from build123d import *

# Parameters (mm, degrees)
ESBO_O1_W                = 20
ESBO_O1_H                = 20
RESSALTO_EXTRUS_O3_DEPTH = 2
CORTE_EXTRUS_O5_DEPTH    = 29.354893758


with BuildPart() as part:
    # Esboço1 → Ressalto-extrusão3 (new body)
    with BuildSketch(Plane(origin=(0, 0, 0), x_dir=(1, 0, 0), z_dir=(0, 1, 0))):
        with Locations((10, 10)):
            Rectangle(ESBO_O1_W, ESBO_O1_H)
    extrude(amount=RESSALTO_EXTRUS_O3_DEPTH)

    # Esboço5 → Corte-extrusão5 (cut, through all)
    with BuildSketch(Plane(origin=(0, 2, 0), x_dir=(1, 0, 0), z_dir=(0, 1, 0))):
        with BuildLine():
            Line((2.309294959, 16.962694399), (2.309294959, 14.191413107))
            ThreePointArc((2.309294959, 14.191413107), (7.109294959, 15.577053753), (2.309294959, 16.962694399))
        make_face()
        with BuildLine():
            Line((2.461667221, 3.455973937), (2.461667221, 6.586469106))
            ThreePointArc((2.461667221, 6.586469106), (7.361667221, 5.021221521), (2.461667221, 3.455973937))
        make_face()
        with BuildLine():
            Line((17.465138281, 14.341379407), (17.465138281, 17.141379407))
            ThreePointArc((17.465138281, 17.141379407), (12.565138281, 15.741379407), (17.465138281, 14.341379407))
        make_face()
        with BuildLine():
            Line((12.486102937, 11.927996301), (12.486102937, 8.765718641))
            ThreePointArc((12.486102937, 8.765718641), (7.486102937, 10.346857471), (12.486102937, 11.927996301))
        make_face()
        with BuildLine():
            Line((17.693873019, 5.738268613), (17.693873019, 2.909841488))
            ThreePointArc((17.693873019, 2.909841488), (12.693873019, 4.32405505), (17.693873019, 5.738268613))
        make_face()
        Polygon((3.125021592, 21.130122811), (-1.51392015, 15.923072084), (-4.183814677, 19.828549229), (-3.382846319, 21.73084908), align=None)
    extrude(amount=-CORTE_EXTRUS_O5_DEPTH, mode=Mode.SUBTRACT)


solid = part.part
Geometry: final body of the model. Coordinates: model frame, mm. A direction names the side the tool comes from. Give positions to 0.01 mm unless a question says otherwise; leave off trailing zeros. Write each loop counter-clockwise with the first axis right and the second up, starting at its lowest first coordinate (ties: lowest second). Pieces come first, ordered by that corner, then holes. Notation, with made-up numbers: (74.5, 46.5) - (131.5, 46.5) arc R21 ccw to (131.5, 59.5) - close; hole circle Ø3 at (72.5, 60.5). An arc over 180 degrees is marked (long way). Return JSON: item names as keys, results as strings. Group by question number.
1) Section A-A on y = 0.4. Return the cut outline in (x, z).
2) Section B-B on z = -13.5. Return the cut outline in (x, y).
3) Section C-C on x = 11. Return the cut outline in (y, z), plus the area to 3 significant figures.
4) Set-up query: faces 1 (the flat face through (12, 0, -8)), 2 (the flat face through (2.309, 1, -16)). Return all of +Z, -Z, +X, -X, +Y, -Y with unobstructed straight access to the full face (end or side cutting, diameter ignored); none if empty.
5) Line query: line 1 (Z direction, x = 4.5, y = 1.35); line 2 (X direction, y = 0.4, z = -3.5); line 3 (Z direction, x = 15.75, y = 0.4). Output: solid intervals per line, ascending.
6) Section D-D on x = 4.25. Return the cut outline in (y, z), plus the area to 3 significant figures.
7) Mould query, pull axis Z, two halves, no side actions, for faces 3 (the flat face through (1.074, 1.014, -18.828)), 4 (the cylindrical face through (7.108, 1.014, -15.483)), 5 (the flat face through (20, 1, -10)). Classes: released by +Z, released by -Z, zero draft, split by the parting line, or undercut.
Filled in:
{
 "1": {"outline": "(0, -17.62) - (2.12, -20) - (20, -20) - (20, 0) - (0, 0) - close; hole (2.31, -16.96) arc R2.6 ccw (long way) to (2.31, -14.19) - close; hole (2.46, -6.59) arc R2.7 ccw (long way) to (2.46, -3.46) - close; hole (12.49, -11.93) - (12.49, -8.77) arc R2.75 ccw (long way) to start; hole (17.47, -17.14) - (17.47, -14.34) arc R2.65 ccw (long way) to start; hole (17.69, -5.74) - (17.69, -2.91) arc R2.7 ccw (long way) to start"},
 "2": {"outline": "(0, 0) - (2.95, 0) - (2.95, 2) - (0, 2) - close; (6.07, 0) - (13.8, 0) - (13.8, 2) - (6.07, 2) - close; (16.63, 0) - (20, 0) - (20, 2) - (16.63, 2) - close"},
 "3": {"outline": "(0, -20) - (2, -20) - (2, -12.99) - (0, -12.99) - close; (0, -7.71) - (2, -7.71) - (2, 0) - (0, 0) - close", "area": "29.4 mm^2"},
 "4": {"face 1": "+Z, -Z, +X, -X, -Y", "face 2": "+Y, -Y"},
 "5": {"line 1": "z = -20 to -18.18, -12.98 to -7.72, -2.33 to 0", "line 2": "x = 0 to 2.46, 6.89 to 12.82, 17.69 to 20", "line 3": "z = -20 to -18.34, -13.15 to -7, -1.65 to 0"},
 "6": {"outline": "(0, -20) - (2, -20) - (2, -18.16) - (0, -18.16) - close; (0, -12.99) - (2, -12.99) - (2, -7.69) - (0, -7.69) - close; (0, -2.35) - (2, -2.35) - (2, 0) - (0, 0) - close", "area": "19.0 mm^2"},
 "7": {"face 3": "released by -Z", "face 4": "undercut", "face 5": "zero draft"}
}
